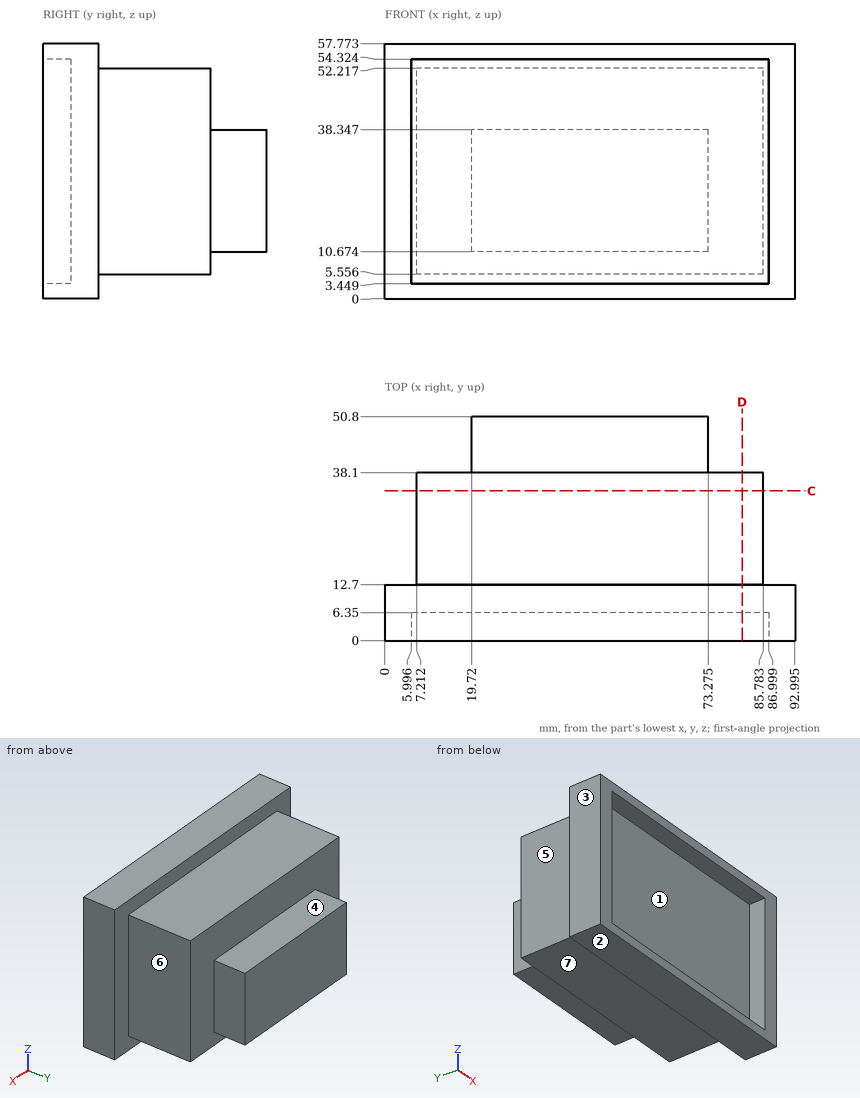
Part print with two shaded views. Sizes in mm from the minimum x, y, z corner. A direction names the side the tool comes from. Coordinates: 2 decimals unless noted, no trailing zeros. Write each loop counter-clockwise with the first axis right and the second up, starting at its lowest first coordinate (ties: lowest second). Pieces come first, ordered by that corner, then holes.
(1) Cut at C-C on y = 34. List the corners of the cut face in (x, z), and give its area (3 significant figures).
(2) Mould opens along X. For the marked faces 1, 2 and 3 say: pulls with the +X half, pulls with the -X half, needs draft (parallel to the pull), parting line crosses it, or undercut.
(3) Cut at D-D on x = 81. List the corners of the cut face in (y, z), and give its area (3 significant figures).
(4) Drill centre lines: line 1 (X direction, y = 3.5, z = 12) (1 decimal); line 2 (Z direction, x = 31.5, y = 45) (1 decimal); line 3 (X direction, y = 20.5, z = 22.5). Where is each one in solid material? Low to high.
(5) 3-axis set-ups, long thin cutter, end or side, ignore diameter. For the marked faces 4, 5, 6 and 7: which of +Z, -Z, +X, -X, +Y, -Y reach the whole face in a straight line?
(6) Pin check, flat tips, straight feed: pin 1 Ø7.5 at (y, z) = (21, 24.5) entering from -X; pin 2 Ø1 at (x, z) = (64, 47.5) entering from +Y; pin 3 Ø6 at (x, y) = (48, 18.5) entering from -Z. Stop position of each tip, or through.
Working result:
1. outline: (7.21, 5.56) - (85.78, 5.56) - (85.78, 52.22) - (7.21, 52.22) - close
1. area: 3,670 mm2
2. face 1: undercut
2. face 2: needs draft
2. face 3: pulls with the -X half
3. outline: (0, 0) - (12.7, 0) - (12.7, 5.56) - (38.1, 5.56) - (38.1, 52.22) - (12.7, 52.22) - (12.7, 57.77) - (0, 57.77) - (0, 54.32) - (6.35, 54.32) - (6.35, 3.45) - (0, 3.45) - close
3. area: 1,600 mm2
4. line 1: x = 0 to 6, 87 to 93
4. line 2: z = 10.7 to 38.3
4. line 3: x = 7.21 to 85.78
5. face 4: +Z, +X, -X, +Y
5. face 5: +Z, -Z, -X, +Y
5. face 6: +Z, -Z, +X, +Y
5. face 7: -Z, +X, -X, +Y
6. pin 1: stops at x = 7.21
6. pin 2: stops at y = 38.1
6. pin 3: stops at z = 5.56
